Autodesk Inventor part; units mm, degrees
ref_plane "YZ Plane" through (0, 0, 0) normal (1, 0, 0) x (0, 1, 0)
ref_plane "XZ Plane" through (0, 0, 0) normal (0, 1, 0) x (-1, 0, 0)
ref_plane "XY Plane" through (0, 0, 0) normal (0, 0, 1) x (1, 0, 0)
sketch "Boceto1" plane through (0, 0, 0) normal (0, 1, 0) x (-1, 0, 0)
  line L0 (0, 0) -> (0, -350)
  line L1 (0, -350) -> (-350, 0)
  line L2 (-350, 0) -> (0, 0)
  dimension "d0" = 350
  dimension "d1" = 45
extrude "Extrusión1" add sketch "Boceto1" along normal blind 1
sketch "Boceto2" plane through (0, 1, 0) normal (0, 1, 0) x (1, 0, 0)
  line L0 (350, 0) -> (0, 350)
  line L1 (174.2929, 174.2929) -> (348.5858, 0)
  line L2 (0, 0) -> (350, 0)
  line L3 (174.2929, 174.2929) -> (420.7803, 174.2929) construction
  line L4 (348.5858, 1) -> (-0.0002, 1)
  line L5 (0, 350) -> (0, 0)
  line L6 (174.2929, 174.2929) -> (0, 348.5858)
  point P0 (347.5858, 1)
  point P1 (0, 1)
  dimension "d5" = 45
  dimension "d6" = 1
  dimension "d7" = 348.586
extrude "Extrusión2" add sketch "Boceto2" along normal blind 348 contours L2 L1 L6 L5 L0 | L2 L5 L4 L1
sketch "Boceto3" plane through (0, 349, 0) normal (0, 1, 0) x (1, 0, 0)
  line L0 (0, 350) -> (0, 0)
  line L1 (0, 0) -> (0, 350)
  line L2 (0, 0) -> (350, 0)
  line L3 (0, 350) -> (350, 0)
  line L4 (350, 0) -> (0, 0)
extrude "Extrusión3" add sketch "Boceto3" along normal blind 1
sketch "Boceto4" plane through (0, 0, -350) normal (-1, 0, 0) x (0, 0, 1)
  point P0 (350, 0)
sketch "Boceto5" plane through (0, 0, -350) normal (-1, 0, 0) x (0, 0, 1)
  line L0 (0, 0) -> (0, 350)
  line L1 (350, 0) -> (0, 0)
  line L2 (0, 0) -> (0, 350)
  line L3 (0, 350) -> (350, 350)
  line L4 (350, 350) -> (350, 0)
  line L5 (349, 1) -> (1.4142, 1)
  line L6 (1.4142, 1) -> (1.4142, 349)
  line L7 (349, 1) -> (1.4142, 1)
  line L8 (1.4142, 1) -> (1.4142, 349)
  line L9 (1.4142, 349) -> (349, 349)
  line L10 (349, 349) -> (349, 1)
extrude "Extrusión4" add sketch "Boceto5" along normal blind 240
sketch "Boceto6" plane through (350, 0, 0) normal (0, 0, 1) x (1, 0, 0)
  line L0 (-590, 0) -> (-590, 350)
  line L1 (-590, 350) -> (-560, 350)
  line L2 (-350, 349) -> (-590, 349)
  line L3 (-590, 350) -> (-560, 350) construction
  line L4 (-560, 350) -> (-560, 332.3)
  line L5 (-590, 0) -> (-560, 0)
  line L6 (-350, 1) -> (-590, 1)
  line L7 (-590, 0) -> (-560, 0) construction
  line L8 (-560, 0) -> (-560, 17.7)
  line L9 (-560, 332.3) -> (-540, 332.3)
  line L10 (-540, 332.3) -> (-540, 17.7)
  line L11 (-540, 17.7) -> (-560, 17.7)
  line L12 (-560, 17.7) -> (-560, 332.3)
  point P0 (-350, 0)
  dimension "d15" = 30
  dimension "d16" = 0
  dimension "d17" = 17.7
  dimension "d18" = 30
  dimension "d19" = 0
  dimension "d20" = 17.7
  dimension "d21" = 90
  dimension "d22" = 20
extrude "Extrusión5" add sketch "Boceto6" along normal blind 25 contours L12 L9 L10 L11
fillet "Empalme1" radius 10 2 edges at (-210, 175, 25) (-190, 175, 25)
sketch "Boceto8" plane through (-210, 332.3, 0) normal (0, 1, 0) x (1, 0, 0)
  line L0 (0, 0) -> (0, -15)
  line L1 (0, -15) -> (10, -15)
  circle A0 centre (10, -15) radius 7
  point P0 (210, 0)
  dimension "d29" = 10
  dimension "d30" = 14
extrude "Extrusión7" cut sketch "Boceto8" against normal blind 1000
properties part number "Cajon_ascensor_mejorsita"
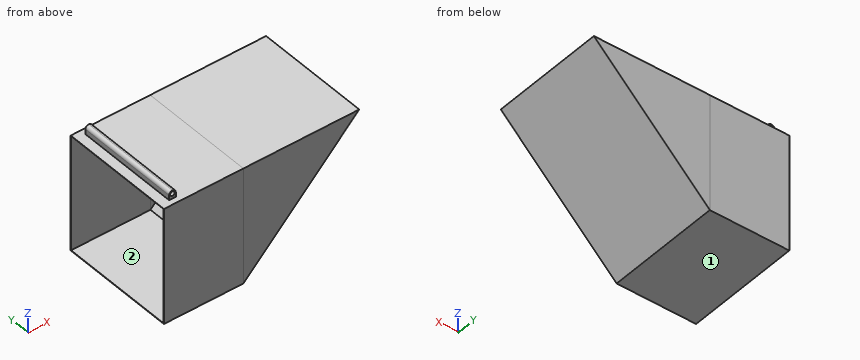
Source: CAD feature listing. Evaluate the final solid. Frame: model axes, mm. Face numbers are marked on the shaded views. Round coordinates to 2 decimals unless told otherwise and drop trailing zeros. Loops run counter-clockwise (first coordinate to the right, second up) from the corner with the lowest first, then second, coordinate; pieces in that order, holes last.
1. Contact query for flat-ended pins moving along their axis: pin 1 (2 mm diameter, centred on y = 161, z = -302.5, fed in from -X); pin 2 (2 mm diameter, centred on y = 210.5, z = -44.5, fed in from -X); pin 3 (4 mm diameter, centred on x = 54, y = 145, fed in from +Z). Output: stop coordinate, or through.
2. Mould query, pull axis Y, two halves, no side actions, for the marked faces 1 and 2. Classes: released by +Y, released by -Y, zero draft, split by the parting line, or undercut.
3. Section query D-D on x = 103.5. Output: boundary loops of the cut face in (y, z).
4. Section query A-A on x = -142. Output: boundary loops of the cut face in (y, z), and give its area (3 significant figures).
5. Section query C-C on z = -111.5. Output: boundary loops of the cut face in (x, y).
6. Ray query, L1, parallel to Z at x = -44, y = 281; L2, parallel to Y at x = 188, z = -17.5; L3, parallel to Z at x = 138, y = 111. Return the intervals inside material, ascending.
Answers below:
1. pin 1: stops at x = 45.09
1. pin 2: stops at x = 303.09
1. pin 3: stops at z = 0
2. face 1: zero draft
2. face 2: undercut
3. outline: (0, -246.5) - (350, -246.5) - (350, 0) - (0, 0) - close; hole (1, -245.09) - (349, -245.09) - (349, -1) - (1, -1) - close
4. outline: (0, -350) - (350, -350) - (350, 0) - (0, 0) - close; hole (1, -348.59) - (349, -348.59) - (349, -1) - (1, -1) - close
4. area: 1,540 mm2
5. outline: (-240, 0) - (238.5, 0) - (238.5, 350) - (-240, 350) - (-240, 349) - (237.09, 349) - (237.09, 1) - (-240, 1) - close
6. L1: z = -350 to -348.59, -1 to 0
6. L2: y = 0 to 1, 349 to 350
6. L3: z = -212 to -210.59, -1 to 0
